from build123d import *

# Parameters (mm, degrees)
SKETCH_1_R      = 6
EXTRUDE_1_DEPTH = 25
M6X1_0_1_D      = 5
M6X1_0_1_DEPTH  = 6
M6X1_0_1_TIP    = 1.502151548
CHAMFER_1_SIZE  = 0.2


with BuildPart() as part:
    # 草图1 → 凸台-拉伸1 (new body)
    with BuildSketch(Plane(origin=(0, 0, 0), x_dir=(1, 0, 0), z_dir=(0, 1, 0))):
        with Locations(Location((0, 0, 0), (0, 0, 270))):
            Circle(SKETCH_1_R)
    extrude(amount=EXTRUDE_1_DEPTH)

    # M6x1.0 螺纹孔1
    with Locations(Plane(origin=(0, 25, 0), x_dir=(1, 0, 0), z_dir=(0, 1, 0))):
        with Locations((0, 0)):
            Hole(M6X1_0_1_D / 2, depth=M6X1_0_1_DEPTH)
            with Locations((0, 0, -(M6X1_0_1_DEPTH + M6X1_0_1_TIP / 2))):  # 118° drill point
                Cone(0, M6X1_0_1_D / 2, M6X1_0_1_TIP, mode=Mode.SUBTRACT)

    # 倒角1
    chamfer_1_edges = [part.edges().sort_by_distance(p)[0] for p in [
        (0, 0, -6),
    ]]
    chamfer(chamfer_1_edges, length=CHAMFER_1_SIZE)


solid = part.part
Read the model definition and answer for the solid it produces. Units are mm, in the model's axes. Round coordinates to 2 decimals unless told otherwise and drop trailing zeros. Loops run counter-clockwise (first coordinate to the right, second up) from the corner with the lowest first, then second, coordinate; pieces in that order, holes last.
Q1. Section A-A on y = 4 is taken. Write down the section's boundary in (x, z).
Q2. Each of these flat-tipped pins is pushed along its axis until it touches: pin 1 (1 mm diameter, centred on x = 2.5, y = 8, fed in from +Z); pin 2 (4 mm diameter, centred on y = 14.5, z = 3.5, fed in from -X); pin 3 (2 mm diameter, centred on x = 2.5, y = 14.5, fed in from -Z). Where does it stop, or does it pass through?
Q3. Determine the mould class of faces 1 (the face through (0.54, 21.96, 2.44)), 2 (the face through (1.802, 12.426, 5.723)), 3 (the face through (0, 0, 0)) for opening direction Z: released by +Z, released by -Z, zero draft, split by the parting line, or undercut.
Q4. Consider probe 1 along Z at (x, y) = (-2, 20); probe 2 along Z at (x, y) = (3.25, 14); probe 3 along Z at (x, y) = (4.5, 9). Determine where each line is inside the solid, lowest interval first.
Output:
1. outline: circle Ø12 at (0, 0)
2. pin 1: stops at z = 5.66
2. pin 2: stops at x = -5.81
2. pin 3: stops at z = -5.81
3. face 1: undercut
3. face 2: split by the parting line
3. face 3: zero draft
4. probe 1: z = -5.66 to -1.5, 1.5 to 5.66
4. probe 2: z = -5.04 to 5.04
4. probe 3: z = -3.97 to 3.97
